Input: part model. Units: mm. Frame: model coordinates. Give positions to 0.01 mm unless a question says otherwise; leave off trailing zeros. Write each loop counter-clockwise with the first axis right and the second up, starting at its lowest first coordinate (ties: lowest second). Pieces come first, ordered by that corner, then holes.
Autodesk Inventor part; units mm, degrees
ref_plane "YZ Plane" through (0, 0, 0) normal (1, 0, 0) x (0, 1, 0)
ref_plane "XZ Plane" through (0, 0, 0) normal (0, 1, 0) x (-1, 0, 0)
ref_plane "XY Plane" through (0, 0, 0) normal (0, 0, 1) x (1, 0, 0)
sketch "Sketch4" plane through (0, 0, 0) normal (0, 1, 0) x (-1, 0, 0)
  circle A0 centre (0, 0) radius 1.5
extrude "Extrusion2" add sketch "Sketch4" along normal mid plane 370
sketch "Sketch13" plane through (0, 0, 0) normal (1, 0, 0) x (0, 1, 0)
  line L0 (185.7937, -0.5) -> (178, -0.5)
  line L1 (178, -0.5) -> (178, -2.4686)
  line L2 (178, -2.4686) -> (185.7937, -2.4686)
  line L3 (185.7937, -2.4686) -> (185.7937, -0.5)
  line L4 (-185, -1.5) -> (185, -1.5)
  line L5 (185, -1.5) -> (185, 1.5)
  line L6 (151, 2.5026) -> (136, 2.5026)
  line L7 (136, 2.5026) -> (136, 0.5)
  line L8 (136, 0.5) -> (151, 0.5)
  line L9 (151, 0.5) -> (151, 2.5026)
  line L10 (-185, 1.5) -> (185, 1.5)
  line L11 (-185, 1.5) -> (-185, -1.5)
  line L12 (3, 4.5) -> (-4, 4.5)
  line L13 (-4, 4.5) -> (-4, 0.5)
  line L14 (-4, 0.5) -> (3, 0.5)
  line L15 (3, 0.5) -> (3, 4.5)
  point P0 (0, 0)
  point P1 (151, 1.5)
  point P2 (136, 1.5)
  point P3 (185, -0.5)
  point P4 (178, -1.5)
  dimension "d89" = 1
  dimension "d90" = 7
  dimension "d91" = 1
  dimension "d92" = 15
  dimension "d96" = 34
  dimension "d97" = 1
  dimension "d98" = 7
  dimension "d99" = 182
extrude "Extrusion9" cut sketch "Sketch13" against normal through all both and the other way through all contours L5 L4 L1 L0 | L9 L8 L7 L10 | L15 L14 L13 L10 | L10 L13 L12 L15
properties part number "Rotating Rod 370mm" material "Bronze, Soft Tin"
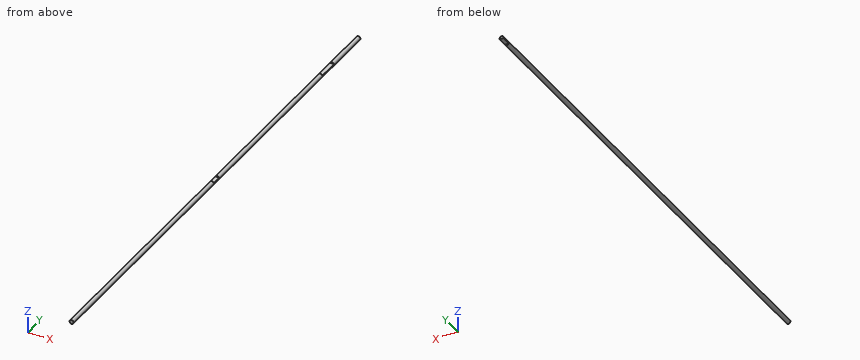
Q1. Pin query (flat end, axial travel): pin 1 (0.8 mm diameter, centred on x = 0, y = 1, fed in from +Z). Return the tip coordinate at first contact, or that it passes through.
Q2. Section B-B, the plane y = -52.5. Return the cut outline in (x, z).
Q3. Section A-A, the plane x = 0. Return the cut outline in (y, z), then the cut area to 3 significant figures.
Q4. Material intervals for line 1 along Y through (x, z) = (-0.1, 1.3); line 2 along Z through (x, y) = (-0.2, 0.5); line 3 along Y through (x, z) = (-0.6, -0.85), sorted ascending.
Solutions:
1. pin 1: stops at z = 0.5
2. outline: circle Ø3 at (0, 0)
3. outline: (-185, -1.5) - (178, -1.5) - (178, -0.5) - (185, -0.5) - (185, 1.5) - (151, 1.5) - (151, 0.5) - (136, 0.5) - (136, 1.5) - (3, 1.5) - (3, 0.5) - (-4, 0.5) - (-4, 1.5) - (-185, 1.5) - close
3. area: 1,080 mm2
4. line 1: y = -185 to -4, 3 to 136, 151 to 185
4. line 2: z = -1.49 to 0.5
4. line 3: y = -185 to 178
